Can you work these out from the drawing? Everything is in mm from the part's minimum corner. Give positions to 0.01 mm unless a question says otherwise; leave off trailing zeros. Order: outer loops, then holes, each group sorted by start corner. A loop starts at its lowest first (then second) coordinate and runs counter-clockwise, first axis right, second up. Notation, with made-up numbers: (51.5, 15) -> (77.5, 15) arc R32 cw to (77.5, 54) -> close; hole circle Ø4 at (-9.5, 27). An arc over 180 degrees is marked (long way). One line per item, written item: value.
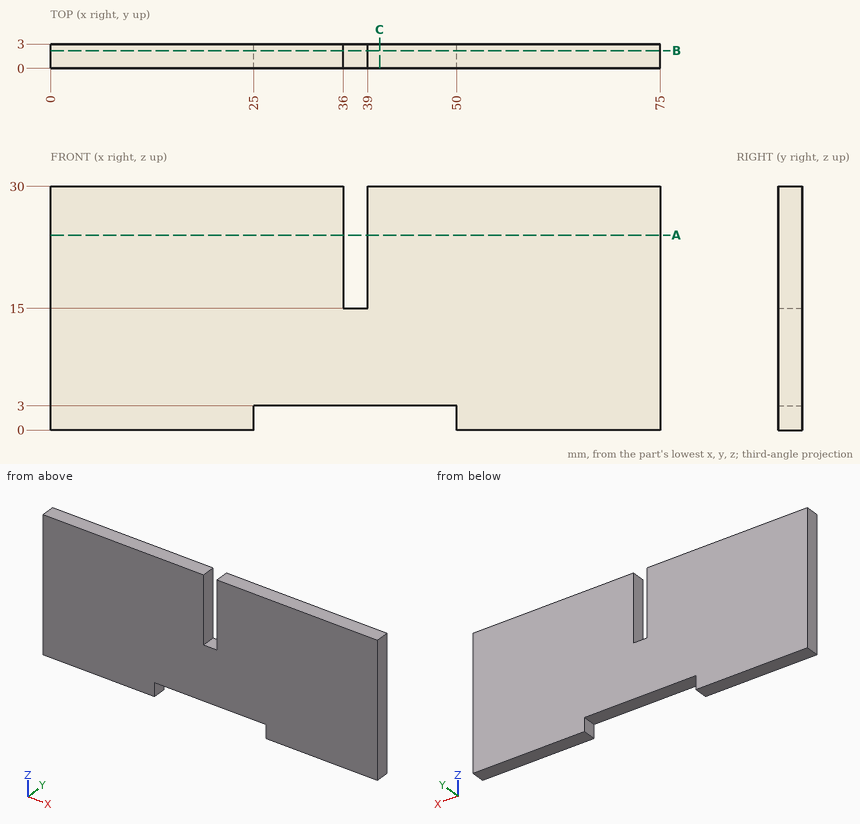
1) Suppose I cut it at A-A, the plane z = 24. Write out the boundary of the cut face in (x, y), then the cut area to 3 significant figures.
Answer below:
outline: (0, 0) -> (36, 0) -> (36, 3) -> (0, 3) -> close; (39, 0) -> (75, 0) -> (75, 3) -> (39, 3) -> close
area: 216 mm2
2) Suppose I cut it at C-C, the plane x = 40.5. Write out the boundary of the cut face in (y, z).
Answer below:
outline: (0, 3) -> (3, 3) -> (3, 30) -> (0, 30) -> close
3) Suppose I cut it at B-B, the plane y = 2.2. Write out the boundary of the cut face in (x, z), then the cut area to 3 significant figures.
Answer below:
outline: (0, 0) -> (25, 0) -> (25, 3) -> (50, 3) -> (50, 0) -> (75, 0) -> (75, 30) -> (39, 30) -> (39, 15) -> (36, 15) -> (36, 30) -> (0, 30) -> close
area: 2,130 mm2
4) If I drill on line 1 along X through (y, z) = (1.25, 22.5); line 2 along Z through (x, y) = (46, 1.95); line 3 along Z through (x, y) = (37, 1.6), over which ranges is the centre line in solid material (lowest first)?
Answer below:
line 1: x = 0 to 36, 39 to 75
line 2: z = 3 to 30
line 3: z = 3 to 15
5) For P1, Ø0.9, axis at y = 1.5, z = 24, coming from the -X side, with a flat end and sliding along its axis, tell me the tip position at first contact or that it passes through.
Answer below:
P1: stops at x = 0
